```python
from build123d import *

# Parameters (mm, degrees)
F0_W          = 609.6
F0_H          = 889
F1_DEPTH      = 12.7
F3_DEPTH      = 25.4
F5_DEPTH      = 25.4
F5_DEPTH_BACK = 114.3
F7_DEPTH      = 101.6


with BuildPart() as f1:
    # F0 (on Top) → F1 (new body)
    with BuildSketch(Plane.XY):
        Rectangle(F0_W, F0_H)
    extrude(amount=F1_DEPTH)

    # F2 (on face) → F3 (join)
    with BuildSketch(Plane.XY.offset(12.7)):
        Polygon((-285.75, -276.225), (-285.75, 276.225), (266.7, 276.225), (266.7, 295.275), (-304.8, 295.275), (-304.8, -295.275), (266.7, -295.275), (266.7, -276.225), align=None)
    extrude(amount=F3_DEPTH)

    # F4 (on face) → F5 (join, two sides)
    with BuildSketch(Plane(origin=(0, 0, 0), x_dir=(1, 0, 0), z_dir=(0, 0, -1))) as f5_sk:
        Polygon((-304.8, 444.5), (304.8, 444.5), (304.8, 463.55), (-323.85, 463.55), (-323.85, -463.55), (304.8, -463.55), (304.8, -444.5), (-304.8, -444.5), align=None)
    extrude(amount=F5_DEPTH)
    extrude(f5_sk.sketch, amount=-F5_DEPTH_BACK)

    # F6 (on face) → F7 (join, through all)
    with BuildSketch(Plane.XY.offset(12.7)):
        Polygon((304.8, -444.5), (304.8, 444.5), (266.7, 444.5), (266.7, 295.275), (266.7, 276.225), (266.7, -276.225), (266.7, -295.275), (266.7, -444.5), align=None)
    extrude(amount=F7_DEPTH)


solid = f1.part
```
Can you work these out from the model? Positions are in its coordinate system, mm. A direction names the side the tool comes from. Coordinates: 2 decimals unless noted, no trailing zeros. Write each loop counter-clockwise with the first axis right and the second up, starting at its lowest first coordinate (ties: lowest second). Pieces come first, ordered by that corner, then holes. Notation, with made-up numbers: M 26,44.25 L 72,44.25 A26 cw 72,71.25 Z; hole C 62,22 d6. An arc over 180 degrees is marked long. Write item = value, one per line. Start each with the question number.
Q1. If we section it at C-C, the plane x = -12.5: Write out the boundary of the cut face in (y, z) (3 decimals).
Q2. On a 3-axis mill with a long thin cutter (end or side, diameter ignored), from which of +Z, -Z, +X, -X, +Y, -Y can I reach the whole of each face in a straight line? I mean faces 1 (the face through (-14, 463.55, 43)), 2 (the face through (-23, 371, 12.7)), 3 (the face through (-4, 6, 0)). Say none if no direction works.
Q3. Thinking about a two-plate mould opening in X: for faces 4 (the face through (-6, -276.225, 25)), 5 (the face through (-304.8, 6, -13)), 6 (the face through (-4, -444.5, -13)), 7 (the face through (-323.85, -6, 43)), which applies, released by +X, released by -X, zero draft, split by the parting line, or undercut?
Q4. I'm going to push flat-ended pins straight in: pin 1 (8 mm diameter, centred on x = -236, y = 45, fed in from -Z); pin 2 (12 mm diameter, centred on x = 98, y = 248, fed in from +Z). Where does each tip first touch, or does it pass through?
Q5. If we section it at B-B, the plane y = 357: Write out the boundary of the cut face in (x, z), then the cut area to 3 significant figures.
Q6. If we section it at A-A, the plane z = 27.5: Write out the boundary of the cut face in (x, y) (3 decimals).
Q7. If we section it at D-D, the plane z = -14.5: Write out the boundary of the cut face in (x, y).
Q8. If I drill on L1, parallel to Y at x = -44.5, z = 36 (3 decimals); L2, parallel to Y at x = 187.5, z = 90; L3, parallel to X at y = -336.5, z = 23, over which ranges is the centre line in solid material (lowest first)? Write a range as [from, to].
Check sheet entries:
q1.outline = M -463.55,-25.4 L -444.5,-25.4 L -444.5,0 L 444.5,0 L 444.5,-25.4 L 463.55,-25.4 L 463.55,114.3 L 444.5,114.3 L 444.5,12.7 L 295.275,12.7 L 295.275,38.1 L 276.225,38.1 L 276.225,12.7 L -276.225,12.7 L -276.225,38.1 L -295.275,38.1 L -295.275,12.7 L -444.5,12.7 L -444.5,114.3 L -463.55,114.3 Z
q2.face_1 = +Z, -Z, +X, -X, +Y
q2.face_2 = +Z
q2.face_3 = -Z, +X
q3.face_4 = undercut
q3.face_5 = released by +X
q3.face_6 = zero draft
q3.face_7 = released by -X
q4.pin_1 = 0
q4.pin_2 = 12.7
q5.outline = M -323.85,-25.4 L -304.8,-25.4 L -304.8,0 L 304.8,0 L 304.8,114.3 L 266.7,114.3 L 266.7,12.7 L -304.8,12.7 L -304.8,114.3 L -323.85,114.3 Z
q5.area = 14,300 mm²
q6.outline = M -323.85,-463.55 L 304.8,-463.55 L 304.8,463.55 L -323.85,463.55 Z; hole M -304.8,-444.5 L 266.7,-444.5 L 266.7,-295.275 L -304.8,-295.275 Z; hole M -304.8,295.275 L 266.7,295.275 L 266.7,444.5 L -304.8,444.5 Z; hole M -285.75,-276.225 L 266.7,-276.225 L 266.7,276.225 L -285.75,276.225 Z
q7.outline = M -323.85,-463.55 L 304.8,-463.55 L 304.8,-444.5 L -304.8,-444.5 L -304.8,444.5 L 304.8,444.5 L 304.8,463.55 L -323.85,463.55 Z
q8.L1 = [-463.55, -444.5], [-295.275, -276.225], [276.225, 295.275], [444.5, 463.55]
q8.L2 = [-463.55, -444.5], [444.5, 463.55]
q8.L3 = [-323.85, -304.8], [266.7, 304.8]
